The listing builds one solid part. Answer for the finished solid, in the listing's coordinates (mm). A direction names the side the tool comes from. Round coordinates to 2 decimals unless told otherwise and drop trailing zeros. Loops run counter-clockwise (first coordinate to the right, second up) from the corner with the lowest first, then second, coordinate; pieces in that order, holes last. Notation, with made-up numbers: (-14, 14.5) - (13, 14.5) arc R20 cw to (13, 43.5) - close; hole circle Ø9 at (22.5, 28). An arc over 180 degrees is marked (long way). One line per question, with ' | ' between items. Start each with the question number.
from build123d import *

# Parameters (mm, degrees)
F0_W      = 23.75
F0_H      = 22
F0_W_2    = 19.75
F0_H_2    = 18
F1_DEPTH  = 2
F2_DEPTH  = 6
F3_W      = 2
F3_H      = 0.5
F4_DEPTH  = 4
F5_DEPTH  = 4
F7_DEPTH  = 6
F8_W      = 3
F8_H      = 4
F9_DEPTH  = 5.2
F10_W     = 0.5
F10_H     = 6
F11_DEPTH = 8
F12_W     = 0.5
F12_H     = 6
F13_DEPTH = 8
F15_DEPTH = 6
F17_DEPTH = 6


# Not quite as in the source:
# - a feature names something its author has since deleted; it is built from what else it names


with BuildPart() as f1:
    # F0 (on Top) → F1 (new body)
    with BuildSketch(Plane.XY):
        Rectangle(F0_W, F0_H)
        Rectangle(F0_W_2, F0_H_2, mode=Mode.SUBTRACT)
        Rectangle(F0_W_2, F0_H_2)
    extrude(amount=F1_DEPTH)

    # F0 (on Top) → F2 (join)
    with BuildSketch(Plane.XY):
        Rectangle(F0_W, F0_H)
        Rectangle(F0_W_2, F0_H_2, mode=Mode.SUBTRACT)
    extrude(amount=F2_DEPTH)

    # F3 (on face) → F4 (cut)
    with BuildSketch(Plane.XY.offset(6)):
        Polygon((10.875, -3), (9.875, -3), (9.875, -3.5), (11.875, -3.5), (11.875, -3), align=None)
        Polygon((9.875, 3.5), (9.875, 3), (10.875, 3), (11.875, 3), (11.875, 3.5), align=None)
        with Locations((-10.875, 3.25)):
            Rectangle(F3_W, F3_H)
        with Locations((-10.875, -3.25)):
            Rectangle(F3_W, F3_H)
    extrude(amount=-F4_DEPTH, mode=Mode.SUBTRACT)

    # F5 (add): faces of the model
    f5_faces = [f1.faces().sort_by_distance(p)[0] for p in [
        (10.875, 0, 6),
        (-10.875, 0, 6),
    ]]
    extrude(f5_faces, amount=F5_DEPTH)

    # F6 (on face) → F7 (join)
    with BuildSketch(Plane.XZ.offset(3)):
        Polygon((11.875, 8), (11.875, 10), (10.375, 8), align=None)
    extrude(amount=-F7_DEPTH)

    # F8 (on face) → F9 (cut)
    with BuildSketch(Plane(origin=(0, 11, 0), x_dir=(-1, 0, 0), z_dir=(0, 1, 0))):
        with Locations((-5.875, 4)):
            Rectangle(F8_W, F8_H)
    extrude(amount=-F9_DEPTH, mode=Mode.SUBTRACT)

    # F10 (on face) → F11 (cut)
    with BuildSketch(Plane.XY.offset(10)):
        with Locations((-10.125, 0)):
            Rectangle(F10_W, F10_H)
    extrude(amount=-F11_DEPTH, mode=Mode.SUBTRACT)

    # F12 (on face) → F13 (cut)
    with BuildSketch(Plane.XY.offset(10)):
        with Locations((10.125, 0)):
            Rectangle(F12_W, F12_H)
    extrude(amount=-F13_DEPTH, mode=Mode.SUBTRACT)

    # F14 (on face) → F15 (join)
    with BuildSketch(Plane.XZ.offset(3)):
        Polygon((10.375, 8), (10.375, 10), (8.875, 8), align=None)
    extrude(amount=-F15_DEPTH)

    # F16 (on face) → F17 (join)
    with BuildSketch(Plane.XZ.offset(3)):
        Polygon((-8.875, 8), (-10.375, 10), (-10.375, 8), align=None)
    extrude(amount=-F17_DEPTH)


solid = f1.part
(1) Determine the mould class of faces 6 (the flat face through (7.375, 10, 4)), 7 (the flat face through (11, 0, 10)), 8 (the flat face through (11.875, 0, 4)) for opening direction X: pulls with the +X half, pulls with the -X half, needs draft (parallel to the pull), parting line crosses it, or undercut.
(2) Consider L1, parallel to Y at x = -10.25, z = 4; L2, parallel to X at y = 0, z = 7.5 (3 decimals); L3, parallel to X at y = 7.25, z = 3 (3 decimals). Determine where each line is inside the solid, lowest interval first.
(3) A tool of negligible diameter and unlimited length cuts with its end or side. For faces 1 (the flat face through (4.375, 10, 4)), 2 (the flat face through (11, -3.5, 4)), 3 (the flat face through (0, -9, 4)), 4 (the flat face through (-10, 0, 8)), 5 (the flat face through (9.636, -0.042, 9.014)), from which of +Z, -Z, +X, -X, +Y, -Y can it reach the whole face along a straight path? Write none if from no direction.
(4) Each of these flat-tipped pins is pushed along its axis until it touches: P1, Ø0.8, axis at x = -10, y = 0, coming from the -Z side; P2, Ø5, axis at x = -5, y = 5.5, coming from the +Z side; P3, Ø6, axis at x = -7.5, y = 5.5, coming from the +Z side; P4, Ø0.9, axis at x = 10, z = 6.5, coming from the -Y side. Where does it stop, or does it pass through?
(5) Find section A-A on z = 4. Write down the section's boundary in (x, y) (3 decimals).
(6) Find section B-B on x = -9.5. Write down the section's boundary in (y, z), plus the area to 3 significant figures.
(7) Find section C-C on y = 4. Write down the section's boundary in (x, z) (3 decimals), plus the area to 3 significant figures.
(8) Find section D-D on z = 7. Write down the section's boundary in (x, y) (3 decimals), plus the area to 3 significant figures.
Answer below:
1) face 6: undercut | face 7: needs draft | face 8: pulls with the +X half
2) L1: -11 to -3.5, 3.5 to 11 | L2: -11.875 to -10.375, 10.375 to 11.875 | L3: -11.875 to -9.875, 9.875 to 11.875
3) face 1: +Z, +Y | face 2: +Z, +X, -X | face 3: +Z | face 4: +Y, -Y | face 5: +Z, +Y, -Y
4) P1: z = 0 | P2: z = 2 | P3: z = 8.38 | P4: y = -3
5) outline: (-11.875, -11) - (11.875, -11) - (11.875, -3.5) - (9.875, -3.5) - (9.875, -9) - (-9.875, -9) - (-9.875, -3.5) - (-11.875, -3.5) - close; (-11.875, -3) - (-10.375, -3) - (-10.375, 3) - (-11.875, 3) - close; (-11.875, 3.5) - (-9.875, 3.5) - (-9.875, 9) - (4.375, 9) - (4.375, 11) - (-11.875, 11) - close; (7.375, 9) - (9.875, 9) - (9.875, 3.5) - (11.875, 3.5) - (11.875, 11) - (7.375, 11) - close; (10.375, -3) - (11.875, -3) - (11.875, 3) - (10.375, 3) - close
6) outline: (-11, 0) - (11, 0) - (11, 6) - (9, 6) - (9, 2) - (-9, 2) - (-9, 6) - (-11, 6) - close; (-3, 8) - (3, 8) - (3, 8.83) - (-3, 8.83) - close | area: 65.0 mm2
7) outline: (-11.875, 0) - (11.875, 0) - (11.875, 6) - (9.875, 6) - (9.875, 2) - (-9.875, 2) - (-9.875, 6) - (-11.875, 6) - close | area: 63.5 mm2
8) outline: (-11.875, -3) - (-10.375, -3) - (-10.375, 3) - (-11.875, 3) - close; (10.375, -3) - (11.875, -3) - (11.875, 3) - (10.375, 3) - close | area: 18.0 mm2
